Build history of the part. All positions in model axes, mm. Face numbers are marked on the shaded views. A direction names the side the tool comes from. Round coordinates to 2 decimals unless told otherwise and drop trailing zeros. Loops run counter-clockwise (first coordinate to the right, second up) from the corner with the lowest first, then second, coordinate; pieces in that order, holes last. Notation, with made-up numbers: (-28, 88) - (-12, 88) arc R21 ccw to (-12, 97) - close; hole circle Ø10 at (80.25, 1). An arc over 180 degrees is marked (long way). Use a Markdown table: item, result.
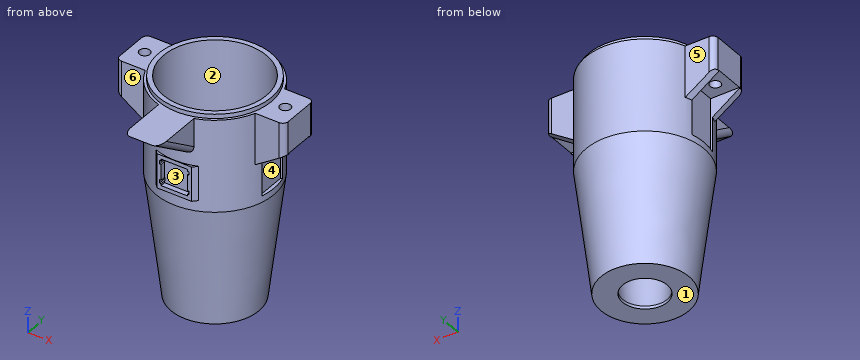
from build123d import *

# Parameters (mm, degrees)
SKETCH1_R               = 13.75
SKETCH1_R_2             = 12
BOSS_EXTRUDE1_DEPTH     = 50
SKETCH2_R               = 1.25
BOSS_EXTRUDE2_DEPTH     = 7.5
SKETCH4_R               = 13.25
BOSS_EXTRUDE3_DEPTH     = 20
SKETCH8_R               = 5.2
CUT_EXTRUDE2_DEPTH      = 20
CHAMFER2_SIZE           = 2.8
CHAMFER2_SIZE2          = 19.311263845
BOSS_EXTRUDE4_DEPTH     = 0.991311543
SKETCH9_W               = 6.2
SKETCH9_H               = 6.2
CUT_EXTRUDE3_DEPTH      = 1.2
CUT_EXTRUDE4_REACH      = 62.367
CUT_EXTRUDE4_END_RADIUS = 12
SKETCH10_W              = 0.5
SKETCH10_H              = 0.8
BOSS_EXTRUDE5_START     = 1
SKETCH11_R              = 13.15
SKETCH11_R_2            = 12
BOSS_EXTRUDE5_DEPTH     = 1
CHAMFER4_SIZE           = 1
SKETCH12_W              = 8.25
SKETCH12_H              = 12
BOSS_EXTRUDE6_DEPTH     = 8.5
CHAMFER5_SIZE           = 8.5
CHAMFER5_SIZE_2         = 12.139258057
FILLET3_R               = 1.5
SKETCH13_W              = 7
SKETCH13_H              = 7
CUT_EXTRUDE5_DEPTH      = 12.5
CHAMFER6_SIZE           = 4.5
CHAMFER6_SIZE_2         = 6.42666603
CHAMFER3_SIZE           = 3.5
CHAMFER3_SIZE2          = 28.505212498
FILLET4_R               = 1.25


with BuildPart() as part:
    # Sketch1 → Boss-Extrude1 (new body)
    with BuildSketch(Plane.XY):
        Circle(SKETCH1_R)
        Circle(SKETCH1_R_2, mode=Mode.SUBTRACT)
    extrude(amount=-BOSS_EXTRUDE1_DEPTH)

    # Sketch2 → Boss-Extrude2 (add)
    # profile 1 of 2: a face of its own
    with BuildSketch(Plane.XY):
        with BuildLine():
            ThreePointArc((-12.808688457, -5), (-13.75, 0), (-12.808688457, 5))
            Line((-12.808688457, 5), (-19.624999957, 5))
            Line((-19.624999957, 5), (-19.624999957, -5))
            Line((-19.624999957, -5), (-12.808688457, -5))
        make_face()
        with Locations((-16.375, 0)):
            Circle(SKETCH2_R, mode=Mode.SUBTRACT)
    # profile 2 of 2: a face of its own
    with BuildSketch(Plane.XY):
        with BuildLine():
            Line((19.624999957, 5), (12.808688457, 5))
            ThreePointArc((12.808688457, 5), (13.512623104, 2.54391762), (13.75, 0))
            ThreePointArc((13.75, 0), (13.512623104, -2.54391762), (12.808688457, -5))
            Line((12.808688457, -5), (19.624999957, -5))
            Line((19.624999957, -5), (19.624999957, 5))
        make_face()
        with Locations((16.375, 0)):
            Circle(SKETCH2_R, mode=Mode.SUBTRACT)
    extrude(amount=-BOSS_EXTRUDE2_DEPTH)

    # Sketch4 → Boss-Extrude3 (add)
    with BuildSketch(Plane(origin=(0, 0, -50), x_dir=(-1, 0, 0), z_dir=(0, 0, -1))):
        Circle(SKETCH4_R)
    extrude(amount=-BOSS_EXTRUDE3_DEPTH)

    # Sketch8 → Cut-Extrude2 (cut)
    with BuildSketch(Plane.XY.offset(-30)):
        Circle(SKETCH8_R)
    extrude(amount=-CUT_EXTRUDE2_DEPTH, mode=Mode.SUBTRACT)

    # Chamfer2
    chamfer2_edges = [part.edges().sort_by_distance(p)[0] for p in [
        (-5.2, 0, -30),
    ]]
    chamfer2_side = [part.faces().sort_by_distance(p)[0] for p in [
        (-11.660588745, 0, -30),
    ]]
    chamfer(chamfer2_edges, length=CHAMFER2_SIZE, length2=CHAMFER2_SIZE2, reference=chamfer2_side[0])

    # 3DSketch3 → Boss-Extrude4 (add)
    with BuildSketch(Plane(origin=(-5, -13.8, -11), x_dir=(0.7808688094430304, 0, -0.6246950475544243), z_dir=(0, -1, 0))):
        Polygon((0, 0), (7.808688094, 6.246950476), (12.806248475, 0), (4.99756038, -6.246950476), align=None)
    extrude(amount=-BOSS_EXTRUDE4_DEPTH)

    # Sketch9 → Cut-Extrude3 (cut)
    with BuildSketch(Plane.XZ.offset(13.8)):
        with Locations((0, -15)):
            Rectangle(SKETCH9_W, SKETCH9_H)
    extrude(amount=-CUT_EXTRUDE3_DEPTH, mode=Mode.SUBTRACT)

    # Cut-Extrude4: up to this cylinder (the profile starts outside it)
    cut_extrude4_end = Plane(origin=(0, 0, -15), z_dir=(0, 0, 1)) * Cylinder(CUT_EXTRUDE4_END_RADIUS, 154.234, mode=Mode.PRIVATE)
    # Sketch10 → Cut-Extrude4 (cut, up to the surface)
    with BuildSketch(Plane.XZ.offset(13.8), mode=Mode.PRIVATE) as cut_extrude4_sk1:
        with Locations((3.2, -12.75)):
            Rectangle(SKETCH10_W, SKETCH10_H)
    cut_extrude4_tool1 = extrude(cut_extrude4_sk1.sketch, amount=-CUT_EXTRUDE4_REACH, mode=Mode.PRIVATE) - cut_extrude4_end
    add(cut_extrude4_tool1.solids().sort_by_distance((3.2, -13.8, -12.75))[0], mode=Mode.SUBTRACT)
    # Sketch10 → Cut-Extrude4 (cut, up to the surface)
    with BuildSketch(Plane.XZ.offset(13.8), mode=Mode.PRIVATE) as cut_extrude4_sk2:
        with Locations((-3.2, -12.75)):
            Rectangle(SKETCH10_W, SKETCH10_H)
    cut_extrude4_tool2 = extrude(cut_extrude4_sk2.sketch, amount=-CUT_EXTRUDE4_REACH, mode=Mode.PRIVATE) - cut_extrude4_end
    add(cut_extrude4_tool2.solids().sort_by_distance((-3.2, -13.8, -12.75))[0], mode=Mode.SUBTRACT)
    # Sketch10 → Cut-Extrude4 (cut, up to the surface)
    with BuildSketch(Plane.XZ.offset(13.8), mode=Mode.PRIVATE) as cut_extrude4_sk3:
        with Locations((3.2, -17.25)):
            Rectangle(SKETCH10_W, SKETCH10_H)
    cut_extrude4_tool3 = extrude(cut_extrude4_sk3.sketch, amount=-CUT_EXTRUDE4_REACH, mode=Mode.PRIVATE) - cut_extrude4_end
    add(cut_extrude4_tool3.solids().sort_by_distance((3.2, -13.8, -17.25))[0], mode=Mode.SUBTRACT)
    # Sketch10 → Cut-Extrude4 (cut, up to the surface)
    with BuildSketch(Plane.XZ.offset(13.8), mode=Mode.PRIVATE) as cut_extrude4_sk4:
        with Locations((-3.2, -17.25)):
            Rectangle(SKETCH10_W, SKETCH10_H)
    cut_extrude4_tool4 = extrude(cut_extrude4_sk4.sketch, amount=-CUT_EXTRUDE4_REACH, mode=Mode.PRIVATE) - cut_extrude4_end
    add(cut_extrude4_tool4.solids().sort_by_distance((-3.2, -13.8, -17.25))[0], mode=Mode.SUBTRACT)

    # Sketch11 → Boss-Extrude5 (add)
    with BuildSketch(Plane.XY.offset(BOSS_EXTRUDE5_START)):
        Circle(SKETCH11_R)
        Circle(SKETCH11_R_2, mode=Mode.SUBTRACT)
    extrude(amount=-BOSS_EXTRUDE5_DEPTH)

    # Chamfer4
    # the kernel refuses this chamfer: 1 mm, written as the material it takes off along each edge
    with BuildSketch(Plane(origin=(-5, -13.8, -21.571682988), x_dir=(0.9996219169112968, -0.027495876610585647, 0), z_dir=(0, 0, 1))) as chamfer4_piece_1_section:
        Polygon((CHAMFER4_SIZE * 0.999621916911, CHAMFER4_SIZE * 0.0274958766106), (-CHAMFER4_SIZE * 0.0274958766106, CHAMFER4_SIZE * 0.999621916911), (0, 0), align=None)
    chamfer4_piece_1 = extrude(amount=13.143365976, mode=Mode.PRIVATE)
    chamfer4_piece_1 = chamfer4_piece_1 - Plane(origin=(0, 0, -15), x_dir=(1, 0, 0), z_dir=(0, 0, 1)) * Cylinder(13.75, 31, mode=Mode.PRIVATE)
    add(chamfer4_piece_1, mode=Mode.SUBTRACT)
    with BuildSketch(Plane(origin=(5, -13.8, -8.428317012), x_dir=(0.02749587661058651, 0.9996219169112968, 0), z_dir=(0, 0, -1))) as chamfer4_piece_2_section:
        Polygon((CHAMFER4_SIZE * 0.999621916911, -CHAMFER4_SIZE * 0.0274958766106), (-CHAMFER4_SIZE * 0.0274958766106, -CHAMFER4_SIZE * 0.999621916911), (0, 0), align=None)
    chamfer4_piece_2 = extrude(amount=13.143365976, mode=Mode.PRIVATE)
    chamfer4_piece_2 = chamfer4_piece_2 - Plane(origin=(0, 0, -15), x_dir=(1, 0, 0), z_dir=(0, 0, 1)) * Cylinder(13.75, 31, mode=Mode.PRIVATE)
    add(chamfer4_piece_2, mode=Mode.SUBTRACT)

    # Sketch12 → Boss-Extrude6 (add)
    with BuildSketch(Plane.XY):
        with Locations((-0.036830357, -19.128189859)):
            Rectangle(SKETCH12_W, SKETCH12_H)
    extrude(amount=-BOSS_EXTRUDE6_DEPTH)

    # Chamfer5
    # the kernel refuses this chamfer: 12.139258057, 8.5 mm, written as the material it takes off along each edge
    with BuildSketch(Plane(origin=(-35.512098327, -25.128189859, -8.5), x_dir=(0, -0.045263737714021236, 0.9989750717851554), z_dir=(1, 0, 0))) as chamfer5_piece_1_section:
        Polygon((CHAMFER5_SIZE * 0.998975071785, -CHAMFER5_SIZE * 0.045263737714), (-CHAMFER5_SIZE_2 * 0.0452637377152, -CHAMFER5_SIZE_2 * 0.998975071811), (0, 0), align=None)
    chamfer5_piece_1 = extrude(amount=70.95053594, mode=Mode.PRIVATE)
    chamfer5_piece_1 = chamfer5_piece_1 - Plane(origin=(0, 0, -5.73810834), x_dir=(1, 0, 0), z_dir=(0, 0, 1)) * Cylinder(13.75, 191, mode=Mode.PRIVATE)
    add(chamfer5_piece_1, mode=Mode.SUBTRACT)

    # Fillet3
    fillet3_edges = [part.edges().sort_by_distance(p)[0] for p in [
        (-4.161830357, -19.128189859, -4.201245229),
        (4.088169643, -19.128189859, -4.201245229),
    ]]
    fillet(fillet3_edges, radius=FILLET3_R)

    # Sketch13 → Cut-Extrude5 (cut)
    with BuildSketch(Plane(origin=(0, 0, -7.5), x_dir=(-1, 0, 0), z_dir=(0, 0, -1))):
        with Locations((-16.375, 0)):
            Rectangle(SKETCH13_W, SKETCH13_H)
        with Locations((16.375, 0)):
            Rectangle(SKETCH13_W, SKETCH13_H)
    extrude(amount=CUT_EXTRUDE5_DEPTH, mode=Mode.SUBTRACT)

    # Chamfer6
    # the kernel refuses this chamfer: 6.42666603, 4.5 mm, written as the material it adds along each edge
    with BuildSketch(Plane(origin=(0, 0, -7.5), x_dir=(-0.008443836697967595, 0.999964350175454, 0), z_dir=(-0.999964350175454, -0.008443836697967595, 0))) as chamfer6_piece_1_section:
        Polygon((13.75, CHAMFER6_SIZE), (13.75 + CHAMFER6_SIZE_2, 0), (13.75, 0), align=None)
    chamfer6_piece_1 = revolve(axis=Axis((0, 0, -7.5), (0, 0, -1)), revolution_arc=144.897264771, mode=Mode.PRIVATE)
    chamfer6_piece_1 = split(chamfer6_piece_1, bisect_by=Plane(origin=(15.287184037, 5, -9.004359876), z_dir=(0, -1, 0)), keep=Keep.TOP, mode=Mode.PRIVATE)
    chamfer6_piece_1 = split(chamfer6_piece_1, bisect_by=Plane(origin=(19.624999957, 4.253690529, -9.004359876), z_dir=(-1, 0, 0)), keep=Keep.TOP, mode=Mode.PRIVATE)
    chamfer6_piece_1 = split(chamfer6_piece_1, bisect_by=Plane(origin=(15.287184037, 3.5, -9.004359876), z_dir=(0, 1, 0)), keep=Keep.TOP, mode=Mode.PRIVATE)
    add(chamfer6_piece_1)
    with BuildSketch(Plane(origin=(0, 0, -7.5), x_dir=(-0.008443836697967595, 0.999964350175454, 0), z_dir=(-0.999964350175454, -0.008443836697967595, 0))) as chamfer6_piece_2_section:
        Polygon((13.75, CHAMFER6_SIZE), (13.75 + CHAMFER6_SIZE_2, 0), (13.75, 0), align=None)
    chamfer6_piece_2 = revolve(axis=Axis((0, 0, -7.5), (0, 0, -1)), revolution_arc=144.897264771, mode=Mode.PRIVATE)
    chamfer6_piece_2 = split(chamfer6_piece_2, bisect_by=Plane(origin=(19.624999957, -4.253690529, -9.004359876), z_dir=(-1, 0, 0)), keep=Keep.TOP, mode=Mode.PRIVATE)
    chamfer6_piece_2 = split(chamfer6_piece_2, bisect_by=Plane(origin=(15.287184037, -3.5, -9.004359876), z_dir=(0, -1, 0)), keep=Keep.TOP, mode=Mode.PRIVATE)
    chamfer6_piece_2 = split(chamfer6_piece_2, bisect_by=Plane(origin=(15.287184037, -5, -9.004359876), z_dir=(0, 1, 0)), keep=Keep.TOP, mode=Mode.PRIVATE)
    add(chamfer6_piece_2)
    with BuildSketch(Plane(origin=(0, 0, -7.5), x_dir=(0.008443836697964339, -0.999964350175454, 0), z_dir=(0.999964350175454, 0.008443836697964339, 0))) as chamfer6_piece_3_section:
        Polygon((13.75, CHAMFER6_SIZE), (13.75 + CHAMFER6_SIZE_2, 0), (13.75, 0), align=None)
    chamfer6_piece_3 = revolve(axis=Axis((0, 0, -7.5), (0, 0, -1)), revolution_arc=144.897264771, mode=Mode.PRIVATE)
    chamfer6_piece_3 = split(chamfer6_piece_3, bisect_by=Plane(origin=(-12.906482524, -5, -11.926294402), z_dir=(0, 1, 0)), keep=Keep.TOP, mode=Mode.PRIVATE)
    chamfer6_piece_3 = split(chamfer6_piece_3, bisect_by=Plane(origin=(-19.624999957, -4.934370219, -11.926294402), z_dir=(1, 0, 0)), keep=Keep.TOP, mode=Mode.PRIVATE)
    chamfer6_piece_3 = split(chamfer6_piece_3, bisect_by=Plane(origin=(-12.906482524, -3.5, -11.926294402), z_dir=(0, -1, 0)), keep=Keep.TOP, mode=Mode.PRIVATE)
    add(chamfer6_piece_3)
    with BuildSketch(Plane(origin=(0, 0, -7.5), x_dir=(0.008443836697964339, -0.999964350175454, 0), z_dir=(0.999964350175454, 0.008443836697964339, 0))) as chamfer6_piece_4_section:
        Polygon((13.75, CHAMFER6_SIZE), (13.75 + CHAMFER6_SIZE_2, 0), (13.75, 0), align=None)
    chamfer6_piece_4 = revolve(axis=Axis((0, 0, -7.5), (0, 0, -1)), revolution_arc=144.897264771, mode=Mode.PRIVATE)
    chamfer6_piece_4 = split(chamfer6_piece_4, bisect_by=Plane(origin=(-19.624999957, 4.25463743, -11.933336397), z_dir=(1, 0, 0)), keep=Keep.TOP, mode=Mode.PRIVATE)
    chamfer6_piece_4 = split(chamfer6_piece_4, bisect_by=Plane(origin=(-13.117325859, 3.5, -11.933336397), z_dir=(0, 1, 0)), keep=Keep.TOP, mode=Mode.PRIVATE)
    chamfer6_piece_4 = split(chamfer6_piece_4, bisect_by=Plane(origin=(-13.117325859, 5, -11.933336397), z_dir=(0, -1, 0)), keep=Keep.TOP, mode=Mode.PRIVATE)
    add(chamfer6_piece_4)

    # Chamfer3
    chamfer3_edges = [part.edges().sort_by_distance(p)[0] for p in [
        (-13.75, 0, -50),
    ]]
    chamfer3_side = [part.faces().sort_by_distance(p)[0] for p in [
        (-13.36109127, 0, -50),
    ]]
    chamfer(chamfer3_edges, length=CHAMFER3_SIZE, length2=CHAMFER3_SIZE2, reference=chamfer3_side[0])

    # Fillet4
    fillet4_edges = [part.edges().sort_by_distance(p)[0] for p in [
        (-19.624999957, -5, -3.75),
        (-19.624999957, 5, -3.75),
        (19.624999957, 5, -3.75),
        (19.624999957, -5, -3.75),
    ]]
    fillet(fillet4_edges, radius=FILLET4_R)


solid = part.part
Q1. Drop flat-ended pins along their axis: pin 1 (12 mm diameter, centred on x = -7.5, z = -31.5, fed in from -Y); pin 2 (1 mm diameter, centred on y = -9.5, z = -40, fed in from -X); pin 3 (1 mm diameter, centred on x = 2, z = -43.5, fed in from -Y). Give the stop position or say it passes through.
Results found:
| item | result |
|---|---|
| pin 1 | stops at y = -12.68 |
| pin 2 | stops at x = -7.13 |
| pin 3 | stops at y = -10.97 |
Q2. Cut at B-B, the plane y = 0. Count the separate pieces of the cut face and the enclosed holes in it, plus the area to 3 significant figures.
Results found:
| item | result |
|---|---|
| separate pieces | 4 |
| enclosed holes | 0 |
| area | 324 mm2 |
Q3. Which spindle directions (+Z, -Z, +X, -X, +Y, -Y) get a long thin tool onto all of the face, cutting with end or side? Do the marked faces 4, 5 and 6. Say none if no direction does.
Results found:
| item | result |
|---|---|
| face 4 | +X |
| face 5 | +Z, -Z, -X, +Y |
| face 6 | +Z, -Z, -X, -Y |
Q4. Cut at D-D, the plane z = -43. List the corners of the cut face in (x, y), plus the area to 3 significant figures.
Results found:
| item | result |
|---|---|
| outline | circle Ø22.22 at (0, 0); hole circle Ø12.23 at (0, 0) |
| area | 270 mm2 |
Q5. Pull direction Z, two halves, no side cores. Call the marked faces 1, 2 and 3: pulls with the +Z half, pulls with the -Z half, needs draft (parallel to the pull), parting line crosses it, or undercut.
Results found:
| item | result |
|---|---|
| face 1 | pulls with the -Z half |
| face 2 | needs draft |
| face 3 | undercut |
Q6. Probe line 1 (Y direction, x = -0.5, z = -28.5); line 2 (Y direction, x = 0, z = -49); line 3 (Z direction, x = 7, y = 4.5). List the from-to ranges inside material, lowest first.
Results found:
| item | result |
|---|---|
| line 1 | y = -12.88 to -11.99, 11.99 to 12.88 |
| line 2 | y = -10.37 to -5.25, 5.25 to 10.37 |
| line 3 | z = -50 to -30 |
